from build123d import *
from build123d.topology import SkipClean

# Parameters (mm, degrees)
SKETCH1_R           = 2.1
BOSS_EXTRUDE1_DEPTH = 3
SKETCH2_R           = 3.9
SKETCH2_R_2         = 2.1
EXTRUDE_THIN1_DEPTH = 7
SKETCH3_W           = 65
SKETCH3_H           = 1
CUT_EXTRUDE1_DEPTH  = 1


with BuildPart() as part:
    # Sketch1 → Boss-Extrude1 (new body)
    with BuildSketch(Plane(origin=(0, 0, 0), x_dir=(1, 0, 0), z_dir=(0, 1, 0))):
        with BuildLine():
            Line((-45, 4), (45, 4))
            ThreePointArc((45, 4), (49, 0), (45, -4))
            Line((45, -4), (-45, -4))
            ThreePointArc((-45, -4), (-49, 0), (-45, 4))
        make_face()
        with Locations(Location((-45, 0, 0), (0, 0, 270))):
            Circle(SKETCH1_R, mode=Mode.SUBTRACT)
        with Locations(Location((45, 0, 0), (0, 0, 270))):
            Circle(SKETCH1_R, mode=Mode.SUBTRACT)
    extrude(amount=-BOSS_EXTRUDE1_DEPTH)

    # Sketch2 → Extrude-Thin1 (add)
    # profile 1 of 2: a face of its own
    with SkipClean():  # the faces are left unmerged after this step: merging them gives an invalid solid
        with BuildSketch(Plane.XZ.offset(3)):
            with Locations((45, 0)):
                Circle(SKETCH2_R)
            with Locations((45, 0)):
                Circle(SKETCH2_R_2, mode=Mode.SUBTRACT)
        # profile 2 of 2: a face of its own
        with BuildSketch(Plane.XZ.offset(3)):
            with Locations((-45, 0)):
                Circle(SKETCH2_R)
            with Locations((-45, 0)):
                Circle(SKETCH2_R_2, mode=Mode.SUBTRACT)
        extrude(amount=EXTRUDE_THIN1_DEPTH)
    add(part.part.scale(1), mode=Mode.REPLACE)  # the faces are merged on a copy

    # Sketch3 → Cut-Extrude1 (cut)
    with BuildSketch(Plane(origin=(0, 0, 0), x_dir=(1, 0, 0), z_dir=(0, 1, 0))):
        Rectangle(SKETCH3_W, SKETCH3_H)
    extrude(amount=-CUT_EXTRUDE1_DEPTH, mode=Mode.SUBTRACT)


solid = part.part
Could you check a few things on this model? Use its own coordinates, in mm. A direction names the side the tool comes from. Give positions to 0.01 mm unless a question says otherwise; leave off trailing zeros. Order: outer loops, then holes, each group sorted by start corner. A loop starts at its lowest first (then second) coordinate and runs counter-clockwise, first axis right, second up.
Item 1: If we section it at C-C, the plane x = -35.5: Write out the boundary of the cut face in (y, z).
Item 2: For faces 1 (the face through (41.104, -6.451, 0.171)), 2 (the face through (1, 0, -1)), which set-ups out of +Z, -Z, +X, -X, +Y, -Y let a thin tool reach every point of the face, with its end or its side?
Item 3: If we section it at B-B, the plane y = -5.75: Write out the boundary of the cut face in (x, z), plus the area to 3 significant figures.
Item 4: I'm going to push flat-ended pins straight in: pin 1 (1.5 mm diameter, centred on y = -7, z = 3, fed in from -X); pin 2 (0.5 mm diameter, centred on x = 12.5, z = 0, fed in from +Y); pin 3 (2.5 mm diameter, centred on x = 17, z = 0, fed in from -Y). Where does each tip first touch, or does it pass through?
Item 5: If we mould it in two halves opening along X, with no side actions, what happens to faces 3 (the face through (1, -3, 0)), 4 (the face through (-1, -1, -4)), 5 (the face through (-49, -1, 0))? For each: pulls with the +X half, pulls with the -X half, needs draft (parallel to the pull), parting line crosses it, or undercut.
Item 6: If we section it at A-A, the plane x = 0: Write out the boundary of the cut face in (y, z), plus the area to 3 significant figures.
Item 7: I need wall thicknesses on line 1 (X direction, y = -0.75, z = 0); line 2 (X direction, y = -6.25, z = 1.5); line 3 (Z direction, x = 45, y = -4.5). Which ranges of each line are inside material? Lowest first, please.
Values:
1. outline: (-3, -4) - (0, -4) - (0, 4) - (-3, 4) - close
2. face 1: -Y
2. face 2: +Z, -Z, +X, -X, +Y
3. outline: circle Ø7.8 at (-45, 0); circle Ø7.8 at (45, 0); hole circle Ø4.2 at (-45, 0); hole circle Ø4.2 at (45, 0)
3. area: 67.9 mm2
4. pin 1: stops at x = -48.19
4. pin 2: stops at y = -1
4. pin 3: stops at y = -3
5. face 3: undercut
5. face 4: needs draft
5. face 5: pulls with the -X half
6. outline: (-3, -4) - (0, -4) - (0, -0.5) - (-1, -0.5) - (-1, 0.5) - (0, 0.5) - (0, 4) - (-3, 4) - close
6. area: 23.0 mm2
7. line 1: x = -49 to -47.1, -42.9 to -32.5, 32.5 to 42.9, 47.1 to 49
7. line 2: x = -48.6 to -46.47, -43.53 to -41.4, 41.4 to 43.53, 46.47 to 48.6
7. line 3: z = -3.9 to -2.1, 2.1 to 3.9
